Here's how the part is built. I have some questions about the finished solid (model axes, mm). Face numbers are marked on the shaded views. Give positions to 0.01 mm unless a question says otherwise; leave off trailing zeros. Order: outer loops, then holes, each group sorted by start corner. A loop starts at its lowest first (then second) coordinate and runs counter-clockwise, first axis right, second up. Notation, with made-up numbers: (37.25, 84.25) -> (44.25, 84.25) arc R11 ccw to (44.25, 93.25) -> close; hole circle Ø4 at (-25.5, -38). An arc over 180 degrees is marked (long way). Write each question's results on one line, items separated by ' | '. Start each with the question number.
Q1. I'm going to push flat-ended pins straight in: pin 1 (6 mm diameter, centred on y = 0, z = 8.27, fed in from -X); pin 2 (6 mm diameter, centred on x = 72.5, z = 2, fed in from +Y); pin 3 (3 mm diameter, centred on y = 9.5, z = -4, fed in from +X); pin 4 (13 mm diameter, centred on y = 0, z = 8.27, fed in from +X). Where does each tip first touch, or does it pass through?
Q2. I need wall thicknesses on line 1 along X through (y, z) = (3, 17); line 2 along Y through (x, z) = (6, -1); line 3 along Y through (x, z) = (70, 11). Which ranges of each line are inside material? Lowest first, please. Write a range as [from, to].
Q3. Imagine slicing it at B-B, the plane x = 30.5. Please give me the cut outline in (y, z).
Q4. Imagine slicing it at A-A, the plane y = 0. Please give me the cut outline in (x, z), then the cut area to 3 significant figures.
Q5. Thinking about a two-plate mould opening in Y: for the marked faces 1, 2 and 3, which applies, pulls with the +Y half, pulls with the -Y half, needs draft (parallel to the pull), parting line crosses it, or undercut?
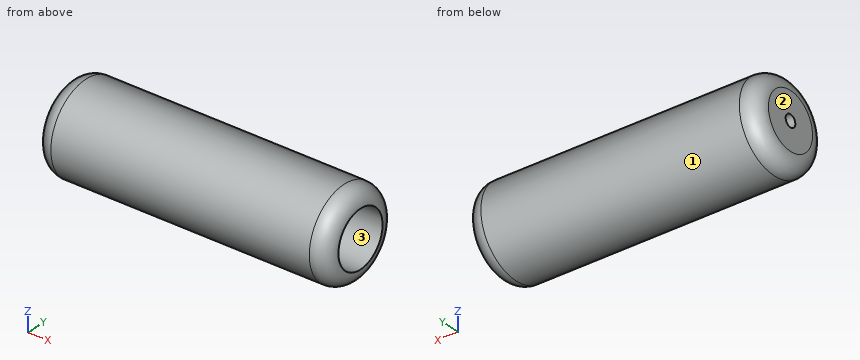
```python
from build123d import *


with BuildPart() as f1:
    # F0 (on Front) → F1 (revolve)
    with BuildSketch(Plane.XZ):
        with BuildLine():
            ThreePointArc((0, -2.6162), (1.859872, -7.106328), (6.35, -8.9662))
            Line((6.35, -8.9662), (107.1626, -8.9662))
            ThreePointArc((107.1626, -8.9662), (111.652728, -7.106328), (113.5126, -2.6162))
            Line((113.5126, -2.6162), (3.9624, -2.6162))
            Line((3.9624, -2.6162), (3.9624, 5.8928))
            Line((3.9624, 5.8928), (0, 5.8928))
            Line((0, 5.8928), (0, -2.6162))
        make_face()
    revolve(axis=Axis((12.4968, 0, 8.27405), (1, 0, 0)))


solid = f1.part
```
Geometry check:
1) pin 1: x = 0 | pin 2: y = 16.93 | pin 3: x = 112.69 | pin 4: x = 3.96
2) line 1: [0, 3.96] | line 2: [-14.52, -5.71], [5.71, 14.52] | line 3: [-17.02, -10.54], [10.54, 17.02]
3) outline: circle Ø34.48 at (0, 8.27); hole circle Ø21.78 at (0, 8.27)
4) outline: (0, -2.62) arc R6.35 ccw to (6.35, -8.97) -> (107.16, -8.97) arc R6.35 ccw to (113.51, -2.62) -> (3.96, -2.62) -> (3.96, 5.89) -> (0, 5.89) -> close; (0, 10.66) -> (3.96, 10.66) -> (3.96, 19.16) -> (113.51, 19.16) arc R6.35 ccw to (107.16, 25.51) -> (6.35, 25.51) arc R6.35 ccw to (0, 19.16) -> close | area: 1,470 mm²
5) face 1: parting line crosses it | face 2: needs draft | face 3: undercut
